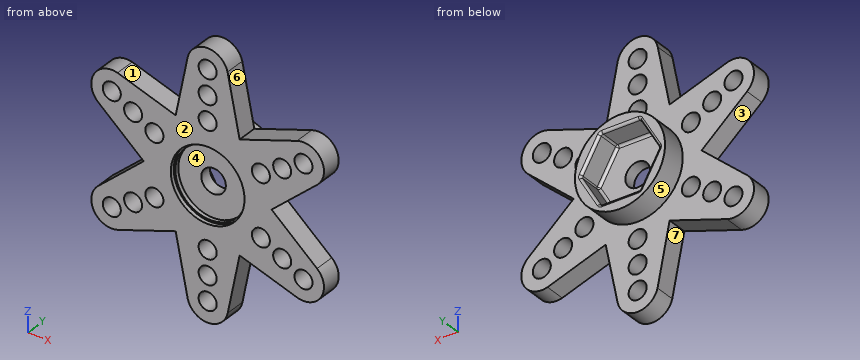
from build123d import *

# Parameters (mm, degrees)
SALIENTE_EXTRUIR1_DEPTH = 2.5
CROQUIS2_R              = 5.5
SALIENTE_EXTRUIR2_DEPTH = 3
CORTAR_EXTRUIR1_REACH   = 7.5
CROQUIS3_R              = 1.5
CROQUIS4_R              = 4.3
CORTAR_EXTRUIR2_DEPTH   = 1
CROQUIS5_R              = 4.5
CROQUIS5_R_2            = 4.3
CORTAR_EXTRUIR3_DEPTH   = 0.5
REDONDEO1_R             = 0.3
CROQUIS6_R              = 1.1
CORTAR_EXTRUIR4_DEPTH   = 2.5
MATRIZC1_COUNT          = 6


with BuildPart() as part:
    # Croquis1 → Saliente-Extruir1 (new body)
    with BuildSketch(Plane(origin=(0, 0, 0), x_dir=(1, 0, 0), z_dir=(0, 1, 0))):
        with BuildLine():
            Line((-3.9, -6.75499815), (-10.994862545, -9.151023749))
            ThreePointArc((-10.994862545, -9.151023749), (-13.88318634, -7.952423618), (-13.342044439, -4.872452504))
            Line((-13.342044439, -4.872452504), (-7.8, 0))
            Line((-7.8, 0), (-13.42245031, 4.9463184))
            ThreePointArc((-13.42245031, 4.9463184), (-13.828594045, 8.046980247), (-10.890689867, 9.11832317))
            Line((-10.890689867, 9.11832317), (-3.9, 6.75499815))
            Line((-3.9, 6.75499815), (-2.427587765, 14.097342149))
            ThreePointArc((-2.427587765, 14.097342149), (0.054592295, 15.999403865), (2.451354572, 13.990775674))
            Line((2.451354572, 13.990775674), (3.9, 6.75499815))
            Line((3.9, 6.75499815), (10.994862545, 9.151023749))
            ThreePointArc((10.994862545, 9.151023749), (13.88318634, 7.952423618), (13.342044439, 4.872452504))
            Line((13.342044439, 4.872452504), (7.8, 0))
            Line((7.8, 0), (13.42245031, -4.9463184))
            ThreePointArc((13.42245031, -4.9463184), (13.828594045, -8.046980247), (10.890689867, -9.11832317))
            Line((10.890689867, -9.11832317), (3.9, -6.75499815))
            Line((3.9, -6.75499815), (2.427587765, -14.097342149))
            ThreePointArc((2.427587765, -14.097342149), (-0.054592295, -15.999403865), (-2.451354572, -13.990775674))
            Line((-2.451354572, -13.990775674), (-3.9, -6.75499815))
        make_face()
    extrude(amount=SALIENTE_EXTRUIR1_DEPTH)

    # Croquis2 → Saliente-Extruir2 (add)
    with BuildSketch(Plane(origin=(0, 2.5, 0), x_dir=(1, 0, 0), z_dir=(0, 1, 0))):
        Circle(CROQUIS2_R)
        Polygon((2.4, -4.156921938), (4.8, 0), (2.4, 4.156921938), (-2.4, 4.156921938), (-4.8, 0), (-2.4, -4.156921938), align=None, mode=Mode.SUBTRACT)
    extrude(amount=SALIENTE_EXTRUIR2_DEPTH)

    # Croquis3 → Cortar-Extruir1 (cut, up to next)
    with BuildSketch(Plane.XZ, mode=Mode.PRIVATE) as cortar_extruir1_sk1:
        Circle(CROQUIS3_R)
    cortar_extruir1_tool1 = extrude(cortar_extruir1_sk1.sketch, amount=-CORTAR_EXTRUIR1_REACH, mode=Mode.PRIVATE) & part.part
    add(cortar_extruir1_tool1.solids().sort_by_distance((0, 0, 0))[0], mode=Mode.SUBTRACT)

    # Croquis4 → Cortar-Extruir2 (cut)
    with BuildSketch(Plane.XZ):
        Circle(CROQUIS4_R)
    extrude(amount=-CORTAR_EXTRUIR2_DEPTH, mode=Mode.SUBTRACT)

    # Croquis5 → Cortar-Extruir3 (cut)
    with BuildSketch(Plane.XZ):
        Circle(CROQUIS5_R)
        Circle(CROQUIS5_R_2, mode=Mode.SUBTRACT)
    extrude(amount=-CORTAR_EXTRUIR3_DEPTH, mode=Mode.SUBTRACT)

    # Redondeo1
    redondeo1_edges = [part.edges().sort_by_distance(p)[0] for p in [
        (0, 2.5, 4.156921938),
        (3.6, 2.5, 2.078460969),
        (3.6, 2.5, -2.078460969),
        (0, 2.5, -4.156921938),
        (-3.6, 2.5, -2.078460969),
        (-3.6, 2.5, 2.078460969),
        (0, 5.5, 4.156921938),
        (2.4, 4, 4.156921938),
        (3.6, 5.5, 2.078460969),
        (4.8, 4, 0),
        (3.6, 5.5, -2.078460969),
        (2.4, 4, -4.156921938),
        (0, 5.5, -4.156921938),
        (-2.4, 4, -4.156921938),
        (-3.6, 5.5, -2.078460969),
        (-4.8, 4, 0),
        (-3.6, 5.5, 2.078460969),
        (-2.4, 4, 4.156921938),
    ]]
    fillet(redondeo1_edges, radius=REDONDEO1_R)

    # Croquis6 → Cortar-Extruir4 (cut)
    with BuildSketch(Plane.XZ):
        with Locations((0, -13.5)):
            Circle(CROQUIS6_R)
        with Locations((0, -10.5)):
            Circle(CROQUIS6_R)
        with Locations((0, -7.5)):
            Circle(CROQUIS6_R)
    cortar_extruir4 = extrude(amount=-CORTAR_EXTRUIR4_DEPTH, mode=Mode.SUBTRACT)

    # MatrizC1: Cortar-Extruir4 ×6 about axis
    matrizc1_axis = Axis((0, 0, 0), (0, 1, 0))
    for i in range(1, MATRIZC1_COUNT):
        add(cortar_extruir4.rotate(matrizc1_axis, i * 360 / MATRIZC1_COUNT), mode=Mode.SUBTRACT)


solid = part.part
Input: part model. Units: mm. Frame: model coordinates. Face numbers are marked on the shaded views. A direction names the side the tool comes from. Give positions to 0.01 mm unless a question says otherwise; leave off trailing zeros. Order: outer loops, then holes, each group sorted by start corner. A loop starts at its lowest first (then second) coordinate and runs counter-clockwise, first axis right, second up. Notation, with made-up numbers: (48.25, 50.5) - (60.25, 50.5) arc R19 cw to (60.25, 83.5) - close; hole circle Ø10 at (-21.5, -10.5). An arc over 180 degrees is marked (long way). Write each question's results on one line, items separated by ' | '.
Item 1: Section D-D (x = 0). Give the number of separate pieces and of enclosed holes in the cut face, and give its area (3 significant figures).
A:
separate pieces: 8 | enclosed holes: 0 | area: 41.8 mm^2
Item 2: Section B-B (z = -10.5). Return loops of the section in (x, y).
A:
outline: (-3.15, 0) - (-1.1, 0) - (-1.1, 2.5) - (-3.15, 2.5) - close; (1.1, 0) - (3.15, 0) - (3.15, 2.5) - (1.1, 2.5) - close
Item 3: Draft query along X for the marked faces 1, 2 and 3. Return one class per face: released by +X, released by -X, zero draft, split by the parting line, or undercut.
A:
face 1: undercut | face 2: zero draft | face 3: released by -X
Item 4: Material intervals for line 1 along Z through (x, y) = (-8.75, 2.25); line 2 along Z through (x, y) = (-9, 1.95); line 3 along X through (y, z) = (3.25, 3.5), sorted ascending.
A:
line 1: z = -8.39 to -6.3, -4.2 to -0.84, 0.84 to 4.2, 6.3 to 8.39 | line 2: z = -8.48 to -6.35, -4.15 to -1.06, 1.06 to 4.15, 6.35 to 8.48 | line 3: x = -4.24 to -2.78, 2.78 to 4.24
Item 5: Contact query for flat-ended pins moving along their axis: pin 1 Ø5 at (x, z) = (0, 0) entering from +Y; pin 2 Ø1 at (y, z) = (4, -4.5) entering from -X; pin 3 Ø2.5 at (x, y) = (0.5, 4.5) entering from -Z. Output: stop coordinate, or through.
A:
pin 1: stops at y = 2.5 | pin 2: stops at x = -3.77 | pin 3: stops at z = -5.5
Item 6: Section A-A (y = 3.25). Return loops of the section in (x, z).
A:
outline: circle Ø11 at (0, 0); hole (-4.71, -0.15) - (-2.49, -4.01) arc R0.3 ccw to (-2.23, -4.16) - (2.23, -4.16) arc R0.3 ccw to (2.49, -4.01) - (4.71, -0.15) arc R0.3 ccw to (4.71, 0.15) - (2.49, 4.01) arc R0.3 ccw to (2.23, 4.16) - (-2.23, 4.16) arc R0.3 ccw to (-2.49, 4.01) - (-4.71, 0.15) arc R0.3 ccw to start
Item 7: Section C-C (x = -6.5). Return loops of the section in (y, z), and give its area (3 significant figures).
A:
outline: (0, -7.63) - (2.5, -7.63) - (2.5, -4.85) - (0, -4.85) - close; (0, -2.65) - (2.5, -2.65) - (2.5, 2.65) - (0, 2.65) - close; (0, 4.85) - (2.5, 4.85) - (2.5, 7.63) - (0, 7.63) - close | area: 27.2 mm^2
Item 8: Access query for the marked faces 4, 5, 6 and 7. Directions: +Z, -Z, +X, -X, +Y, -Y. A direction counts if a zero-diameter tool reaches every point of the face in a straight line with its end or side. Return the directions, or none.
A:
face 4: -Y | face 5: +Y | face 6: +Z, +Y, -Y | face 7: -Z, +Y, -Y
